from build123d import *

# Parameters (mm, degrees)
F0_R     = 22.5
F1_DEPTH = 150
F1_TAPER = -3
F2_T     = -2.5
F3_R     = 1.75
F4_DEPTH = 6
F4_TAPER = 5


with BuildPart() as f1:
    # F0 (on Top) → F1 (new body)
    with BuildSketch(Plane.XY):
        Circle(F0_R)
    extrude(amount=F1_DEPTH, taper=F1_TAPER)

    # F2
    f2_openings = [f1.faces().sort_by_distance(p)[0] for p in [
        (0, 0, 150),
    ]]
    offset(amount=F2_T, openings=f2_openings, kind=Kind.INTERSECTION)

    # F3 (on Top) → F4 (join)
    with BuildSketch(Plane.XY):
        Circle(F3_R)
    extrude(amount=-F4_DEPTH, taper=F4_TAPER)


solid = f1.part
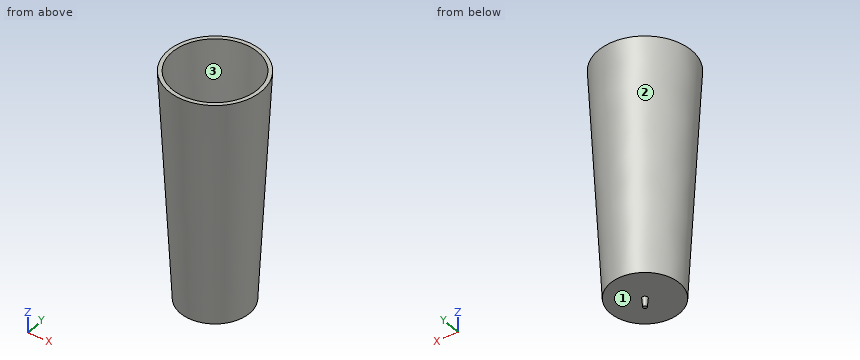
Here's how the part is built. I have some questions about the finished solid (model axes, mm). Face numbers are marked on the shaded views. Give positions to 0.01 mm unless a question says otherwise; leave off trailing zeros. Loops run counter-clockwise (first coordinate to the right, second up) from the corner with the lowest first, then second, coordinate; pieces in that order, holes last. Notation, with made-up numbers: (66.5, -12) -> (86.5, -12) arc R11 ccw to (86.5, 0) -> close; hole circle Ø11 at (53, 6.25). An arc over 180 degrees is marked (long way). Answer as a JSON object with one key per item and string values. Group by question number.
Item 1: I need wall thicknesses on L1, parallel to X at y = -6, z = 33; L2, parallel to Y at x = -4, z = 21.5; L3, parallel to X at y = -9.5, z = 51. Which ranges of each line are inside material? Lowest first, please.
Item 2: Thinking about a two-plate mould opening in X: for the marked faces 1, 2 and 3, which applies, pulls with the +X half, pulls with the -X half, needs draft (parallel to the pull), parting line crosses it, or undercut?
Item 3: Imagine slicing it at B-B on z = 30. Write out the boundary of the cut face in (x, y), then the cut area to 3 significant figures.
Item 4: Will these pins go through, and if not, where does the flat tip stop? pin 1 (1.5 mm diameter, centred on y = -17, z = 60, fed in from +X); pin 2 (6 mm diameter, centred on x = -8.5, z = 94.5, fed in from +Y); pin 3 (6 mm diameter, centred on y = 3.5, z = 49.5, fed in from -X).
Item 5: Imagine slicing it at A-A on z = 132. Write out the boundary of the cut face in (x, y), then the cut area to 3 significant figures.
Answer list:
{
 "1": {"L1": "x = -23.47 to -20.88, 20.88 to 23.47", "L2": "y = -23.29 to -20.74, 20.74 to 23.29", "L3": "x = -23.31 to -20.58, 20.58 to 23.31"},
 "2": {"face 1": "needs draft", "face 2": "parting line crosses it", "face 3": "undercut"},
 "3": {"outline": "circle Ø48.14 at (0, 0); hole circle Ø43.14 at (0, 0)", "area": "359 mm2"},
 "4": {"pin 1": "stops at x = 19.84", "pin 2": "stops at y = 26.92", "pin 3": "stops at x = -25.17"},
 "5": {"outline": "circle Ø58.84 at (0, 0); hole circle Ø53.83 at (0, 0)", "area": "443 mm2"}
}
